Design review of the part shown in the three views and the two pictorial views. Dimensions are in mm from the part's minimum x, y and z. Give positions to 0.01 mm unless a question says otherwise; leave off trailing zeros. Loops run counter-clockwise (first coordinate to the right, second up) from the corner with the lowest first, then second, coordinate; pieces in that order, holes last.
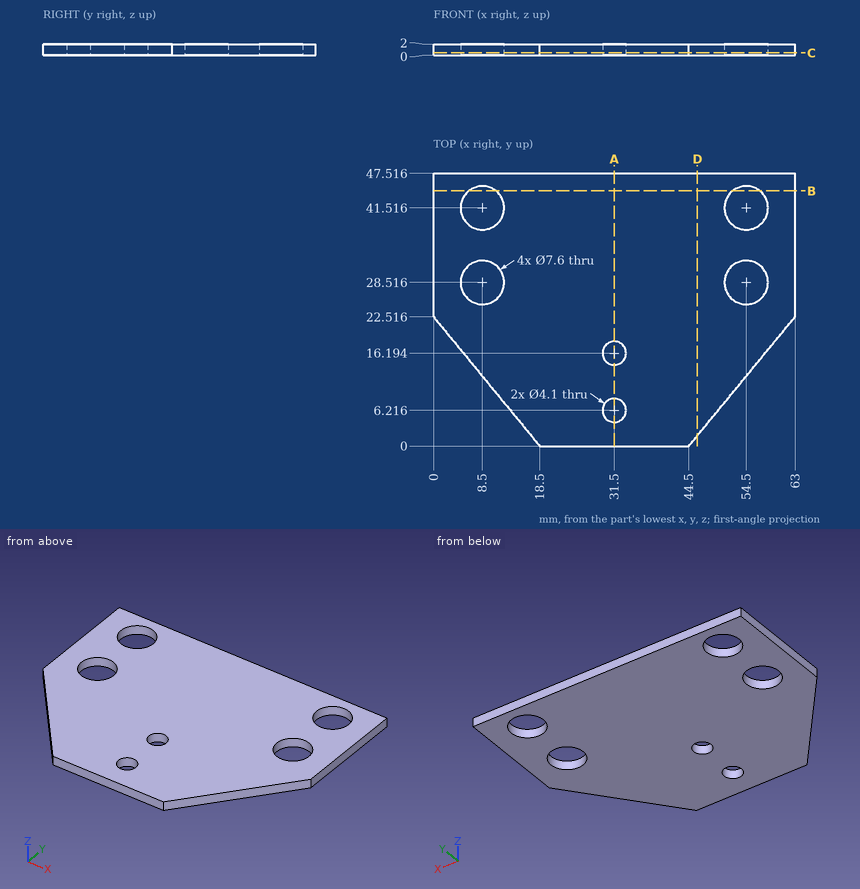
Q1. Consider section B-B on y = 44.5. Give the boundary of the cut face in (x, z).
Answers:
outline: (0, 0) - (6.15, 0) - (6.15, 2) - (0, 2) - close; (10.85, 0) - (52.15, 0) - (52.15, 2) - (10.85, 2) - close; (56.85, 0) - (63, 0) - (63, 2) - (56.85, 2) - close
Q2. Consider section D-D on x = 46. Give the boundary of the cut face in (y, z) (1 decimal).
Answers:
outline: (1.8, 0) - (47.5, 0) - (47.5, 2) - (1.8, 2) - close
Q3. Consider section C-C on z = 0.45. Count the separate pieces of the cut face and the enclosed holes in it, plus the area to 3 significant figures.
Answers:
separate pieces: 1
enclosed holes: 6
area: 2,370 mm2
Q4. For pin 1 Ø4.5 at (x, y) = (54.5, 28.52) entering from +Z; pin 2 Ø4.5 at (x, y) = (31.5, 16.19) entering from -Z; pin 3 Ø1 at (y, z) = (19, 0.5) entering from +X, all flat-tipped, find the tip position at first contact; note any pin that passes through.
Answers:
pin 1: passes through
pin 2: stops at z = 0
pin 3: stops at x = 60.52
Q5. For probe 1 along Y at (x, z) = (31.5, 0.95) (1 decimal); probe 2 along Y at (x, z) = (53, 0.7) (1 decimal); probe 3 along X at (y, z) = (29, 1.8), list the stretches that pass through material, from the lowest coordinate up.
Answers:
probe 1: y = 0 to 4.2, 8.3 to 14.1, 18.2 to 47.5
probe 2: y = 10.3 to 25, 32 to 38, 45 to 47.5
probe 3: x = 0 to 4.73, 12.27 to 50.73, 58.27 to 63
Q6. Consider section A-A on x = 31.5. Give the boundary of the cut face in (y, z) (1 decimal).
Answers:
outline: (0, 0) - (4.2, 0) - (4.2, 2) - (0, 2) - close; (8.3, 0) - (14.1, 0) - (14.1, 2) - (8.3, 2) - close; (18.2, 0) - (47.5, 0) - (47.5, 2) - (18.2, 2) - close
